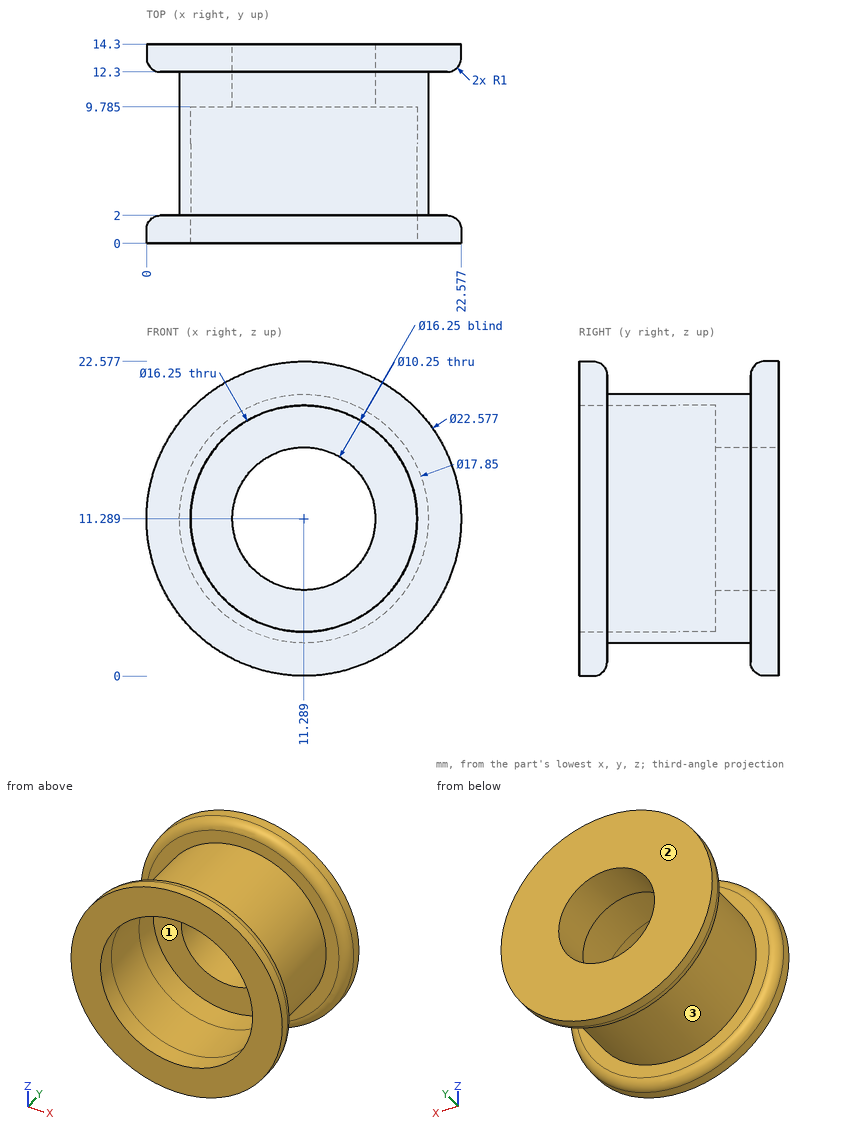
Verification items for this drawing (mm, ordinates from the low corner). Round coordinates to 2 decimals unless told otherwise and drop trailing zeros. Write item = value, one per line. Start each with the question number.
1) Gauge pin test, flat ends, axial feed: pin 1 Ø2 at (y, z) = (10, 4.5) entering from +X; pin 2 Ø9 at (x, z) = (11.29, 11.29) entering from -Y. Record the tip position at first contact, or that the pin passes through.
2) Thickness scan on probe 1 along Y at (x, z) = (19.75, 7.5); probe 2 along X at (y, z) = (11.5, 11.5); probe 3 along X at (y, z) = (12, 14.5) (1 decimal). Record the ranges inside material, lowest first.
3) Release check for a two-part mould opening along X. For the marked faces 1, 2 and 3 record: released by +X, released by -X, zero draft, split by the parting line, or undercut.
Results are:
q1.pin_1 = 18.08
q1.pin_2 = through
q2.probe_1 = 0 to 2, 12.3 to 14.3
q2.probe_2 = 2.37 to 6.17, 16.41 to 20.21
q2.probe_3 = 3 to 7.3, 15.3 to 19.6
q3.face_1 = undercut
q3.face_2 = zero draft
q3.face_3 = split by the parting line
